Source: CAD feature listing. Evaluate the final solid. Frame: model axes, mm. Face numbers are marked on the shaded views. Coordinates: 2 decimals unless noted, no trailing zeros. Order: outer loops, then holes, each group sorted by start corner. A loop starts at its lowest first (then second) coordinate and runs counter-clockwise, first axis right, second up.
Item 1: Mould query, pull axis X, two halves, no side actions, for the marked faces 1, 2 and 3. Classes: released by +X, released by -X, zero draft, split by the parting line, or undercut.
Item 2: Section A-A on y = 41. Return the cut outline in (x, z).
Item 3: Contact query for flat-ended pins moving along their axis: P1, Ø6, axis at x = -13, z = -13, coming from the -Y side; P2, Ø1, axis at x = 11.5, z = 2, coming from the +Y side; P3, Ø4, axis at y = 114, z = -3.5, coming from the -X side; P4, Ø3.5, axis at x = 0, z = 0, coming from the -Y side. Output: stop coordinate, or through.
Item 4: Ray query, line 1 (Z direction, x = 0, y = 132.55); line 2 (Y direction, x = 7.5, z = -17). Return the intervals inside material, ascending.
Autodesk Inventor part; units mm, degrees
ref_plane "YZ Plane" through (0, 0, 0) normal (1, 0, 0) x (0, 1, 0)
ref_plane "XZ Plane" through (0, 0, 0) normal (0, 1, 0) x (-1, 0, 0)
ref_plane "XY Plane" through (0, 0, 0) normal (0, 0, 1) x (1, 0, 0)
sketch "Sketch1" plane through (0, 0, 0) normal (0, 1, 0) x (-1, 0, 0)
  circle A0 centre (0, 0) radius 16.5
  line L0 (0, -23.5) -> (18, -23.5)
  line L1 (18, -9.261) -> (18, 9.261)
  line L2 (-18, 9.261) -> (-18, -9.261)
  line L3 (-18, -23.5) -> (18, 23.5) construction
  line L4 (18, -23.5) -> (-18, 23.5) construction
  arc A1 (18, 9.261) -> (-18, 9.261) centre (0, 5.0033) ccw
  line L5 (28.3506, 0) -> (-36.241, 0) construction
  arc A2 (-18, -9.261) -> (18, -9.261) centre (0, -5.0033) ccw
  circle A3 centre (0, 0) radius 17.5
  dimension "d0" = 33
  dimension "d1" = 36
  dimension "d2" = 47
  dimension "d3" = 1
extrude "Extrusion1" add sketch "Sketch1" along normal blind 115 contours A3
extrude "Extrusion2" add sketch "Sketch1" along normal blind 3
sketch "Sketch2" plane through (0, 0, 0) normal (0, 0, 1) x (1, 0, 0)
  line L0 (16.5, 3) -> (16.5, 115)
  line L1 (16.5, 115) -> (11, 115)
  line L2 (17.5, 115) -> (-17.5, 115)
  line L3 (11, 115) -> (6.2224, 118.6297)
  line L4 (6.2224, 118.6297) -> (3.2708, 127.1319)
  line L5 (3.2708, 127.1319) -> (4.2154, 127.4599)
  line L6 (4.2154, 127.4599) -> (9.99, 118.6297)
  line L7 (17.5, 115) -> (16.6596, 116.8149)
  line L8 (16.6596, 116.8149) -> (9.99, 118.6297)
  line L9 (3.2708, 127.1319) -> (1.9591, 130.9102)
  line L10 (1.9591, 130.9102) -> (2.3904, 131.1923)
  line L11 (2.3904, 131.1923) -> (4.2154, 127.4599)
  line L12 (1.9591, 130.9102) -> (1.9591, 133.9102)
  line L13 (1.9591, 133.9102) -> (2.3904, 133.9102)
  line L14 (2.3904, 133.9102) -> (2.3904, 131.1923)
  line L15 (0, -26.782) -> (0, 160.6923)
  point P0 (0, 0)
  dimension "d8" = 5.5
  dimension "d9" = 6
  dimension "d10" = 9
  dimension "d11" = 1
  dimension "d12" = 2
  dimension "d13" = 3
revolve "Revolution1" add sketch "Sketch2" angle 360 about axis through (0, -10, 0) along (0, 1, 0)
extrude "Extrusion3" cut sketch "Sketch1" along normal blind 1 contours A0
properties part number "Larger Syringe"
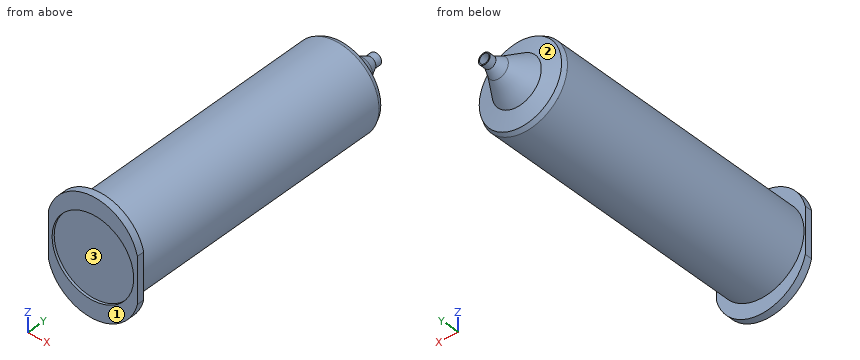
Answer list:
1. face 1: zero draft
1. face 2: split by the parting line
1. face 3: undercut
2. outline: circle Ø35 at (0, 0); hole circle Ø33 at (0, 0)
3. P1: stops at y = 0
3. P2: stops at y = 118.31
3. P3: stops at x = -17.44
3. P4: stops at y = 1
4. line 1: z = -2.39 to -1.96, 1.96 to 2.39
4. line 2: y = 0 to 3
